The listing builds one solid part. Answer for the finished solid, in the listing's coordinates (mm). Face numbers are marked on the shaded views. A direction names the side the tool comes from. Coordinates: 2 decimals unless noted, no trailing zeros. Write each loop counter-clockwise with the first axis right and the second up, starting at its lowest first coordinate (ties: lowest second). Pieces come first, ordered by that corner, then holes. Notation, with made-up numbers: M -7,16 L 26,16 A26 cw 26,51 Z; hole C 60.25,87 d7. An arc over 180 degrees is marked long. Answer as a JSON object with one key per item and string values. Group by question number.
from build123d import *

# Parameters (mm, degrees)
SKETCH3_R             = 46
SKETCH3_R_2           = 3.5
BOSS_EXTRUDE2_DEPTH   = 20
FILLET1_R             = 1
SKETCH4_R             = 12
BOSS_EXTRUDE3_DEPTH   = 10
SKETCH5_R             = 33
CUT_EXTRUDE1_DEPTH    = 14
SKETCH6_R             = 2.5
CUT_EXTRUDE2_DEPTH    = 6
SKETCH7_R             = 7
CUT_EXTRUDE3_DEPTH    = 10
CHAMFER1_SIZE         = 1
CHAMFER1_SIZE2        = 1.732050808
CHAMFER1_PART_2_SIZE  = 1
CHAMFER1_PART_2_SIZE2 = 1.732050808
SKETCH8_R             = 4
CUT_EXTRUDE4_DEPTH    = 47.0000001


with BuildPart() as part:
    # Sketch3 → Boss-Extrude2 (new body)
    with BuildSketch(Plane(origin=(0, 0, 0), x_dir=(1, 0, 0), z_dir=(0, 1, 0))):
        Circle(SKETCH3_R)
        with Locations((0, 36)):
            Circle(SKETCH3_R_2, mode=Mode.SUBTRACT)
        with Locations((31.176914536, 18)):
            Circle(SKETCH3_R_2, mode=Mode.SUBTRACT)
        with Locations((31.176914536, -18)):
            Circle(SKETCH3_R_2, mode=Mode.SUBTRACT)
        with Locations((0, -36)):
            Circle(SKETCH3_R_2, mode=Mode.SUBTRACT)
        with Locations((-31.176914536, -18)):
            Circle(SKETCH3_R_2, mode=Mode.SUBTRACT)
        with Locations((-31.176914536, 18)):
            Circle(SKETCH3_R_2, mode=Mode.SUBTRACT)
    extrude(amount=BOSS_EXTRUDE2_DEPTH)

    # Fillet1
    fillet1_edges = [part.edges().sort_by_distance(p)[0] for p in [
        (-46, 20, 0),
    ]]
    fillet(fillet1_edges, radius=FILLET1_R)

    # Sketch4 → Boss-Extrude3 (add)
    with BuildSketch(Plane(origin=(0, 20, 0), x_dir=(1, 0, 0), z_dir=(0, 1, 0))):
        Circle(SKETCH4_R)
    extrude(amount=BOSS_EXTRUDE3_DEPTH)

    # Sketch5 → Cut-Extrude1 (cut)
    with BuildSketch(Plane.XZ):
        Circle(SKETCH5_R)
    extrude(amount=-CUT_EXTRUDE1_DEPTH, mode=Mode.SUBTRACT)

    # Sketch6 → Cut-Extrude2 (cut)
    with BuildSketch(Plane.XZ.offset(-14)):
        Circle(SKETCH6_R)
    extrude(amount=-CUT_EXTRUDE2_DEPTH, mode=Mode.SUBTRACT)

    # Sketch7 → Cut-Extrude3 (cut)
    with BuildSketch(Plane(origin=(0, 30, 0), x_dir=(1, 0, 0), z_dir=(0, 1, 0))):
        Circle(SKETCH7_R)
    extrude(amount=-CUT_EXTRUDE3_DEPTH, mode=Mode.SUBTRACT)

    # Chamfer1
    chamfer1_edges = [part.edges().sort_by_distance(p)[0] for p in [
        (-7, 20, 0),
    ]]
    chamfer1_side = [part.faces().sort_by_distance(p)[0] for p in [
        (-7, 25, 0),
    ]]
    chamfer(chamfer1_edges, length=CHAMFER1_SIZE, length2=CHAMFER1_SIZE2, reference=chamfer1_side[0])

    # Chamfer1 part 2
    chamfer1_part_2_edges = [part.edges().sort_by_distance(p)[0] for p in [
        (-7, 30, 0),
    ]]
    chamfer1_part_2_side = [part.faces().sort_by_distance(p)[0] for p in [
        (-11.660588745, 30, 0),
    ]]
    chamfer(chamfer1_part_2_edges, length=CHAMFER1_PART_2_SIZE, length2=CHAMFER1_PART_2_SIZE2, reference=chamfer1_part_2_side[0])

    # Sketch8 → Cut-Extrude4 (cut, through all)
    with BuildSketch(Plane(origin=(0, 0, 0), x_dir=(0, 0, -1), z_dir=(1, 0, 0))):
        with Locations((0, 8)):
            Circle(SKETCH8_R)
    extrude(amount=CUT_EXTRUDE4_DEPTH, mode=Mode.SUBTRACT)


solid = part.part
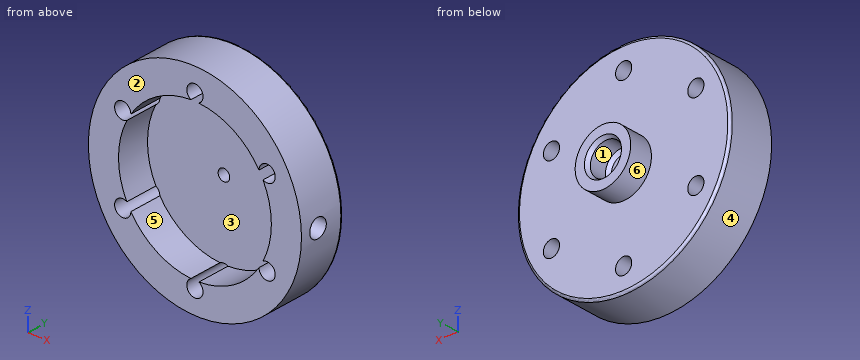
Item 1: For a pull along Z with two mould halves and no side action, classify the marked faces 1, 2, 3 and 4 as +Z half, -Z half, draft (parallel to the pull), parting line (faces both ways), or undercut.
Item 2: Flat-ended cylindrical pins translate along their axes: pin 1 Ø12 at (x, z) = (13, -18) entering from +Y; pin 2 Ø4.5 at (x, z) = (0, 0) entering from +Y; pin 3 Ø18 at (x, z) = (0, 0) entering from -Y; pin 4 Ø1.5 at (y, z) = (5.5, -23) entering from -X. Find the tip coordinate at first contact, or state that the pin passes through.
Item 3: A tool of negligible diameter and unlimited length cuts with its end or side. For the marked faces 5 and 6, from which of +Z, -Z, +X, -X, +Y, -Y can it reach the whole face along a straight path? Write none if from no direction.
Item 4: Consider L1, parallel to Z at x = -33.5, y = 1.5; L2, parallel to Y at x = -14, z = 12.5; L3, parallel to X at y = 7, z = -18.5. Determine where each line is inside the solid, lowest interval first. Write a range as from..to.
Item 5: A cutting plane is placed at C-C, the plane y = 23.5. Write down the section's boundary in (x, z), and give its area (3 significant figures).
Item 6: A cutting plane is placed at B-B, the plane y = 16.5. Write down the section's boundary in (x, z), and give its area (3 significant figures).
Item 7: A cutting plane is placed at A-A, the plane x = 0. State how many separate pieces and enclosed holes the cut face has, and give its area (3 significant figures).
Answer:
{
 "1": {"face 1": "undercut", "face 2": "draft", "face 3": "undercut", "face 4": "parting line"},
 "2": {"pin 1": "y = 20", "pin 2": "through", "pin 3": "y = 14", "pin 4": "x = -40.26"},
 "3": {"face 5": "-Y", "face 6": "+Y"},
 "4": {"L1": "-31.52..-20.62, -15.38..15.38, 20.62..31.52", "L2": "14..20", "L3": "-42.12..-34.64, -27.71..-27.33, 27.33..27.71, 34.64..42.12"},
 "5": {"outline": "C 0,0 d24; hole C 0,0 d14", "area": "298 mm2"},
 "6": {"outline": "C 0,0 d92; hole C -31.18,-18 d7; hole C -31.18,18 d7; hole C 0,-36 d7; hole C 0,36 d7; hole C 0,0 d5; hole C 31.18,-18 d7; hole C 31.18,18 d7", "area": "6,400 mm2"},
 "7": {"separate pieces": "4", "enclosed holes": "0", "area": "720 mm2"}
}
